Verification items for the finished model (mm, model axes). A direction names the side the tool comes from. Give positions to 0.01 mm unless a question says otherwise; leave off trailing zeros. Order: outer loops, then holes, each group sorted by start corner. A loop starts at its lowest first (then second) coordinate and runs counter-clockwise, first axis right, second up. Notation, with made-up numbers: M 72.5,-14 L 107.5,-14 A23 cw 107.5,-2 Z; hole C 82.5,-6.5 d10. An arc over 180 degrees is marked long. Answer as a JSON object with one key per item and string values.
```python
from build123d import *

# Parameters (mm, degrees)
BOSS_EXTRUDE1_DEPTH          = 1.5875
SKETCH7_W                    = 1.5875
SKETCH7_H                    = 101.6
BOSS_EXTRUDE2_DEPTH          = 0.0254
EDGE_FLANGE1_STRIP_W         = 19.05
EDGE_FLANGE1_STRIP_H         = 1.5875
EDGE_FLANGE1_STRIP_CUT_DEPTH = 101.6
EDGE_FLANGE1_DEPTH           = 101.6
SKETCH11_W                   = 101.6
SKETCH11_H                   = 1.5875
BOSS_EXTRUDE3_DEPTH          = 0.0254
EDGE_FLANGE2_STRIP_W         = 19.05
EDGE_FLANGE2_STRIP_H         = 1.5875
EDGE_FLANGE2_STRIP_CUT_DEPTH = 101.6
EDGE_FLANGE2_DEPTH           = 101.6
SKETCH15_R                   = 3.175
CUT_EXTRUDE1_DEPTH           = 2.54
SKETCH16_R                   = 3.175
CUT_EXTRUDE2_DEPTH           = 2.54
CUT_EXTRUDE4_DEPTH           = 2.54


# Sheet-metal steps are written as plain solids
with BuildPart() as part:
    # Sketch1 → Boss-Extrude1 (new body)
    with BuildSketch(Plane.XY):
        Polygon((0, 119.481843199), (0, -32.918156801), (152.4, -32.918156801), align=None)
    extrude(amount=BOSS_EXTRUDE1_DEPTH)

    # Sketch7 → Boss-Extrude2 (add)
    with BuildSketch(Plane.ZY):
        with Locations((0.79375, 43.281843199)):
            Rectangle(SKETCH7_W, SKETCH7_H)
    extrude(amount=BOSS_EXTRUDE2_DEPTH)

    # Edge-Flange1 strip (across the edge) → Edge-Flange1 strip cut (cut)
    with BuildSketch(Plane(origin=(-0.0254, 94.081843199, 1.5875), x_dir=(1, 0, 0), z_dir=(0, -1, 0))):
        with Locations((-1.5875, -0.79375)):
            Rectangle(EDGE_FLANGE1_STRIP_W, EDGE_FLANGE1_STRIP_H)
    extrude(amount=EDGE_FLANGE1_STRIP_CUT_DEPTH, mode=Mode.SUBTRACT)

    # Edge-Flange1 section (across the edge) → Edge-Flange1 (add)
    with BuildSketch(Plane(origin=(-0.0254, 94.081843199, 1.5875), x_dir=(1, 0, 0), z_dir=(0, -1, 0))):
        with BuildLine():
            Line((0, 6.35), (0, 23.8125))
            Line((0, 23.8125), (1.5875, 23.8125))
            Line((1.5875, 23.8125), (1.5875, 6.35))
            ThreePointArc((1.5875, 6.35), (3.447371939, 1.859871939), (7.9375, 0))
            Line((7.9375, 0), (7.9375, -1.5875))
            ThreePointArc((7.9375, -1.5875), (2.324839924, 0.737339924), (0, 6.35))
        make_face()
    extrude(amount=EDGE_FLANGE1_DEPTH)

    # Sketch11 → Boss-Extrude3 (add)
    with BuildSketch(Plane(origin=(0, -32.918156801, 0), x_dir=(-1, 0, 0), z_dir=(0, -1, 0))):
        with Locations((-76.2, -0.79375)):
            Rectangle(SKETCH11_W, SKETCH11_H)
    extrude(amount=BOSS_EXTRUDE3_DEPTH)

    # Edge-Flange2 strip (across the edge) → Edge-Flange2 strip cut (cut)
    with BuildSketch(Plane(origin=(25.4, -32.943556801, 1.5875), x_dir=(0, 1, 0), z_dir=(1, 0, 0))):
        with Locations((-1.5875, -0.79375)):
            Rectangle(EDGE_FLANGE2_STRIP_W, EDGE_FLANGE2_STRIP_H)
    extrude(amount=EDGE_FLANGE2_STRIP_CUT_DEPTH, mode=Mode.SUBTRACT)

    # Edge-Flange2 section (across the edge) → Edge-Flange2 (add)
    with BuildSketch(Plane(origin=(25.4, -32.943556801, 1.5875), x_dir=(0, 1, 0), z_dir=(1, 0, 0))):
        with BuildLine():
            Line((0, 6.35), (0, 23.8125))
            Line((0, 23.8125), (1.5875, 23.8125))
            Line((1.5875, 23.8125), (1.5875, 6.35))
            ThreePointArc((1.5875, 6.35), (3.447371939, 1.859871939), (7.9375, 0))
            Line((7.9375, 0), (7.9375, -1.5875))
            ThreePointArc((7.9375, -1.5875), (2.324839924, 0.737339924), (0, 6.35))
        make_face()
    extrude(amount=EDGE_FLANGE2_DEPTH)

    # Sketch15 → Cut-Extrude1 (cut)
    with BuildSketch(Plane(origin=(0, -31.356056801, 0), x_dir=(1, 0, 0), z_dir=(0, 1, 0))):
        with Locations(Location((38.1, -19.05, 0), (0, 0, 270))):
            Circle(SKETCH15_R)
        with Locations(Location((63.5, -19.05, 0), (0, 0, 270))):
            Circle(SKETCH15_R)
        with Locations(Location((88.9, -19.05, 0), (0, 0, 270))):
            Circle(SKETCH15_R)
        with Locations(Location((114.3, -19.05, 0), (0, 0, 270))):
            Circle(SKETCH15_R)
    extrude(amount=-CUT_EXTRUDE1_DEPTH, mode=Mode.SUBTRACT)

    # Sketch16 → Cut-Extrude2 (cut)
    with BuildSketch(Plane(origin=(1.5621, 0, 0), x_dir=(0, 0, -1), z_dir=(1, 0, 0))):
        with Locations((-19.05, 81.381843199)):
            Circle(SKETCH16_R)
        with Locations((-19.05, 55.981843199)):
            Circle(SKETCH16_R)
        with Locations((-19.05, 30.581843199)):
            Circle(SKETCH16_R)
        with Locations((-19.05, 5.181843199)):
            Circle(SKETCH16_R)
    extrude(amount=-CUT_EXTRUDE2_DEPTH, mode=Mode.SUBTRACT)

    # Sketch17 → Cut-Extrude4 (cut)
    with BuildSketch(Plane(origin=(0, 0, 0), x_dir=(-1, 0, 0), z_dir=(0, 0, -1))):
        with BuildLine():
            add(Edge.make_bspline(
                [(-18.559829118, -11.912329653), (-18.517563518, -11.616470453), (-18.438315518, -11.030035253), (-18.401333118, -10.734176053)],
                knots=[0, 0, 0, 0, 1, 1, 1, 1], degree=3))
            add(Edge.make_bspline(
                [(-18.401333118, -10.734176053), (-18.691909118, -2.819942453), (-17.418657918, 5.120707147), (-18.602094718, 12.950409547)],
                knots=[0, 0, 0, 0, 1, 1, 1, 1], degree=3))
            add(Edge.make_bspline(
                [(-18.602094718, 12.950409547), (-20.817014275, 19.201191532), (-25.977441918, 23.238769538)],
                knots=[0, 0, 0, 1, 1, 1], degree=2))
            Line((-25.977441918, 23.238769538), (-25.977441918, 41.725320732))
            Line((-25.977441918, 41.725320732), (-35.509588786, 41.725320732))
            Line((-35.509588786, 41.725320732), (-35.509588786, 26.702452856))
            add(Edge.make_bspline(
                [(-35.509588786, 26.702452856), (-40.874741805, 27.199220364), (-43.710628887, 23.238769538)],
                knots=[0, 0, 0, 1, 1, 1], degree=2))
            Line((-43.710628887, 23.238769538), (-43.710628887, 39.06666413))
            Line((-43.710628887, 39.06666413), (-51.873392585, 39.06666413))
            Line((-51.873392585, 39.06666413), (-51.873392585, 23.238769538))
            add(Edge.make_bspline(
                [(-51.873392585, 23.238769538), (-54.008947234, 28.015586517), (-59.291846155, 27.844961118)],
                knots=[0, 0, 0, 1, 1, 1], degree=2))
            Line((-59.291846155, 27.844961118), (-59.291846155, 41.800648781))
            Line((-59.291846155, 41.800648781), (-64.561793613, 41.800648781))
            Line((-64.561793613, 41.800648781), (-64.561793613, 27.844961118))
            add(Edge.make_bspline(
                [(-75.385928318, 19.427612747), (-71.900151449, 25.9887548), (-64.561793613, 27.844961118)],
                knots=[0, 0, 0, 1, 1, 1], degree=2))
            Line((-75.385928318, 19.427612747), (-74.810059518, -5.762684853))
            Line((-74.810059518, -5.762684853), (-66.341089918, -7.315945653))
            Line((-66.341089918, -7.315945653), (-56.281940787, -9.411792826))
            Line((-56.281940787, -9.411792826), (-56.281940787, -1.261313945))
            Line((-56.281940787, -1.261313945), (-59.291846155, -0.609067129))
            Line((-59.291846155, -0.609067129), (-59.291846155, 12.950409547))
            add(Edge.make_bspline(
                [(-59.291846155, 12.950409547), (-54.000334372, 11.743104523), (-52.999057908, 6.165627848)],
                knots=[0, 0, 0, 1, 1, 1], degree=2))
            Line((-52.999057908, 6.165627848), (-52.999057908, -1.972715017))
            Line((-52.999057908, -1.972715017), (-52.999057908, -10.095789128))
            Line((-52.999057908, -10.095789128), (-38.803453862, -13.053476327))
            Line((-38.803453862, -13.053476327), (-38.803453862, -5.048903937))
            Line((-38.803453862, -5.048903937), (-41.596172219, -4.44372157))
            Line((-41.596172219, -4.44372157), (-41.596172219, 11.108656065))
            ThreePointArc((-41.596172219, 11.108656065), (-38.214050979, 13.096353593), (-35.509588786, 10.254598891))
            Line((-35.509588786, 10.254598891), (-35.509588786, -5.762684853))
            Line((-35.509588786, -5.762684853), (-35.509588786, -13.734915973))
            Line((-35.509588786, -13.734915973), (-25.977441918, -15.610569653))
            add(Edge.make_bspline(
                [(-25.977441918, -15.610569653), (-23.166779518, -16.720041653), (-19.611185918, -15.261878453), (-18.628510718, -12.408950453)],
                knots=[0, 0, 0, 0, 1, 1, 1, 1], degree=3))
            Line((-18.628510718, -12.408950453), (-18.559829118, -11.912329653))
        make_face()
    extrude(amount=-CUT_EXTRUDE4_DEPTH, mode=Mode.SUBTRACT)


solid = part.part
```
Q1. Material ranges on L1, parallel to X at y = -31.75, z = 19.05 (3 decimals); L2, parallel to Y at x = 0.5, z = 19.05; L3, parallel to Z at x = 45, y = 54.5, recorded low to high.
Resolved:
{"L1": "x = 25.4 to 34.925, 41.275 to 60.325, 66.675 to 85.725, 92.075 to 111.125, 117.475 to 127", "L2": "y = -7.52 to 2.01, 8.36 to 27.41, 33.76 to 52.81, 59.16 to 78.21, 84.56 to 94.08", "L3": "z = 0 to 1.59"}
Q2. Release check for a two-part mould opening along Y. For faces 6 (the face through (1.562, 44, 17)), 7 (the face through (75, -32.944, 17)), 8 (the face through (0.779, 78.282, 19.738)), 9 (the face through (2.361, 43.993, 2.263)) record: +Y half, -Y half, draft (parallel to the pull), parting line (faces both ways), or undercut.
Resolved:
{"face 6": "draft", "face 7": "-Y half", "face 8": "undercut", "face 9": "undercut"}
Q3. Section check A-A on z = 12.75. Record the cut outline in (x, y).
Resolved:
{"outline": "M -0.03,-7.52 L 1.56,-7.52 L 1.56,94.08 L -0.03,94.08 Z; M 25.4,-32.94 L 127,-32.94 L 127,-31.36 L 25.4,-31.36 Z"}
Q4. Gauge pin test, flat ends, axial feed: pin 1 Ø0.8 at (y, z) = (-6, 1) entering from +X; pin 2 Ø1.3 at (y, z) = (-27.5, 1) entering from -X; pin 3 Ø10 at (y, z) = (82.5, 3) entering from +X. Record the tip position at first contact, or that the pin passes through.
Resolved:
{"pin 1": "stops at x = 125.88", "pin 2": "stops at x = 0", "pin 3": "stops at x = 41.78"}
Q5. Tool access check on faces 1 (the face through (25.4, -32, 13)), 2 (the face through (127, -32, 13)), 3 (the face through (0.78, 33.73, 19.46)), 4 (the face through (75, -31.356, 17)), 5 (the face through (1, -7.518, 13)). Record the directions out of +Z, -Z, +X, -X, +Y, -Y that give a thin tool (end or side, any length) a straight path to the whole face; none if there is none.
Resolved:
{"face 1": "+Z, -X, +Y, -Y", "face 2": "+Z, +X, +Y, -Y", "face 3": "+X, -X", "face 4": "+Z, +X, -X, +Y", "face 5": "+Z, +X, -X, -Y"}
